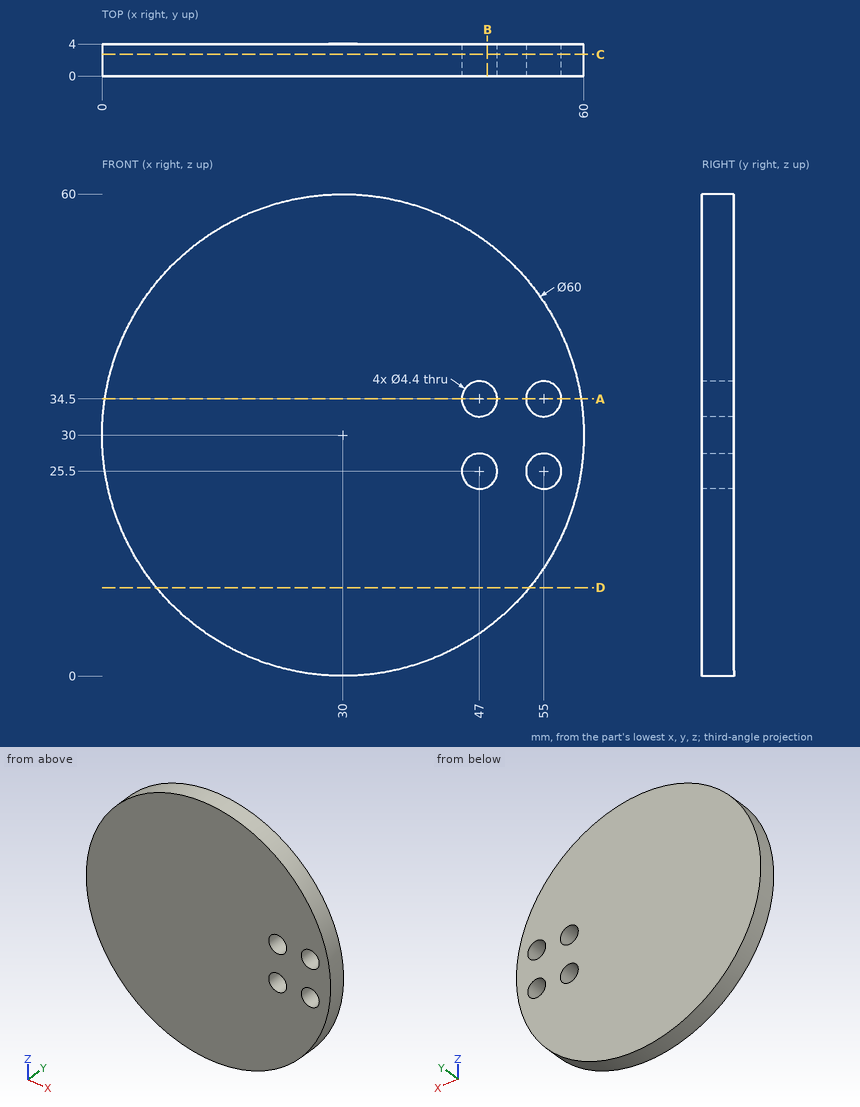
Design review of the part shown in the three views and the two pictorial views. Dimensions are in mm from the part's minimum x, y and z. Coordinates: 2 decimals unless noted, no trailing zeros. Write each loop counter-clockwise with the first axis right and the second up, starting at its lowest first coordinate (ties: lowest second). Pieces come first, ordered by that corner, then holes. Notation, with made-up numbers: (-21.75, 35) - (27.25, 35) arc R28 cw to (27.25, 64) - close; hole circle Ø2 at (0.5, 39.5). An arc over 180 degrees is marked (long way). Write item = value, one per line.
(1) For P1, Ø1, axis at x = 34, y = 2.5, coming from the -Z side; P2, Ø2, axis at y = 1, z = 40, coming from the +X side, all flat-tipped, find the tip position at first contact; note any pin that passes through.
Result sheet:
P1 = 0.2
P2 = 58.62
(2) Consider section A-A, the plane z = 34.5. Give the boundary of the cut face in (x, y).
Result sheet:
outline = (0.34, 0) - (44.8, 0) - (44.8, 4) - (0.34, 4) - close; (49.2, 0) - (52.8, 0) - (52.8, 4) - (49.2, 4) - close; (57.2, 0) - (59.66, 0) - (59.66, 4) - (57.2, 4) - close
(3) Consider section D-D, the plane z = 11. Give the boundary of the cut face in (x, y).
Result sheet:
outline = (6.78, 0) - (53.22, 0) - (53.22, 4) - (6.78, 4) - close
(4) For line 1 (Z direction, x = 47, y = 3.15); line 2 (Z direction, x = 54, y = 3.5); line 3 (X direction, y = 1.7, z = 7), list the stretches that pass through material, from the lowest coordinate up. Write a range as [from, to].
Result sheet:
line_1 = [5.28, 23.3], [27.7, 32.3], [36.7, 54.72]
line_2 = [12, 23.54], [27.46, 32.54], [36.46, 48]
line_3 = [10.74, 49.26]
(5) Consider section C-C, the plane y = 2.7. Give the boundary of the cut face in (x, z), then the cut area to 3 significant figures.
Result sheet:
outline = circle Ø60 at (30, 30); hole circle Ø4.4 at (47, 25.5); hole circle Ø4.4 at (47, 34.5); hole circle Ø4.4 at (55, 25.5); hole circle Ø4.4 at (55, 34.5)
area = 2,770 mm^2
(6) Consider section B-B, the plane x = 48. Give the boundary of the cut face in (y, z), then the cut area to 3 significant figures.
Result sheet:
outline = (0, 6) - (4, 6) - (4, 23.54) - (0, 23.54) - close; (0, 27.46) - (4, 27.46) - (4, 32.54) - (0, 32.54) - close; (0, 36.46) - (4, 36.46) - (4, 54) - (0, 54) - close
area = 161 mm^2
